Could you check a few things on this model? Use its own coordinates, in mm. Face numbers are marked on the shaded views. A direction names the side the tool comes from. Coordinates: 2 decimals unless noted, no trailing zeros. Loops run counter-clockwise (first coordinate to the right, second up) from the corner with the lowest first, then second, coordinate; pieces in that order, holes last. Notation, with made-up numbers: M 39,67 L 61,67 A21 cw 61,98 Z; hole C -20.5,-34 d5. An arc over 180 degrees is marked long. Write each question's results on one line, items separated by ' | '.
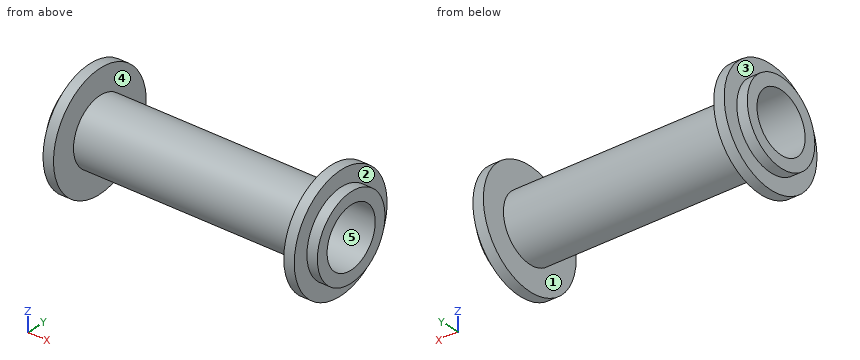
```python
from build123d import *

# Parameters (mm, degrees)
SKETCH2_R           = 5.7
CUT_EXTRUDE1_DEPTH  = 51.457903246
SKETCH3_R           = 8
SKETCH3_R_2         = 5.7
BOSS_EXTRUDE1_DEPTH = 2
SKETCH4_R           = 8
SKETCH4_R_2         = 5.7
BOSS_EXTRUDE2_DEPTH = 2


with BuildPart() as part:
    # Sketch1 → Revolve1 (revolve)
    with BuildSketch(Plane.XY, mode=Mode.PRIVATE) as revolve1_sk:
        Polygon((-24, 0), (24, 0), (24, 11), (22, 11), (22, 6.25), (-22, 6.25), (-22, 11), (-24, 11), align=None)
    revolve(revolve1_sk.sketch.rotate(Axis((-24, 0, 0), (1, 0, 0)), 180), axis=Axis((-24, 0, 0), (1, 0, 0)))

    # Sketch2 → Cut-Extrude1 (cut, through all)
    with BuildSketch(Plane(origin=(24, 0, 0), x_dir=(0, 0, -1), z_dir=(1, 0, 0))):
        Circle(SKETCH2_R)
    extrude(amount=-CUT_EXTRUDE1_DEPTH, mode=Mode.SUBTRACT)

    # Sketch3 → Boss-Extrude1 (add)
    with BuildSketch(Plane(origin=(24, 0, 0), x_dir=(0, 0, -1), z_dir=(1, 0, 0))):
        with Locations(Location((0, 0, 0), (0, 0, 270))):
            Circle(SKETCH3_R)
        Circle(SKETCH3_R_2, mode=Mode.SUBTRACT)
    extrude(amount=BOSS_EXTRUDE1_DEPTH)

    # Sketch4 → Boss-Extrude2 (add)
    with BuildSketch(Plane.ZY.offset(24)):
        with Locations(Location((0, 0, 0), (0, 0, 270))):
            Circle(SKETCH4_R)
        with Locations(Location((0, 0, 0), (0, 0, 180))):
            Circle(SKETCH4_R_2, mode=Mode.SUBTRACT)
    extrude(amount=BOSS_EXTRUDE2_DEPTH)


solid = part.part
```
(1) Will these pins go through, and if not, where does the flat tip stop? P1, Ø1, axis at x = -10, y = -5, coming from the -Z side; P2, Ø8, axis at x = -7, z = -6, coming from the +Y side; P3, Ø8, axis at x = -9.5, z = 7.5, coming from the +Y side.
Reported:
P1: stops at z = -4.34 | P2: stops at y = 5.92 | P3: stops at y = 5.18
(2) Imagine slicing it at C-C, the plane x = -15. List the corners of the cut face in (y, z) for me, and give its area (3 significant figures).
Reported:
outline: C 0,0 d12.5; hole C 0,0 d11.4 | area: 20.6 mm2
(3) Please list where these lines run through material, in increasing order: probe 1 along Z at (x, y) = (4, 0); probe 2 along X at (y, z) = (7.5, -3.5); probe 3 along Y at (x, z) = (-15, -0.5). Write a range as from..to.
Reported:
probe 1: z = -6.25..-5.7, 5.7..6.25 | probe 2: x = -24..-22, 22..24 | probe 3: y = -6.23..-5.68, 5.68..6.23
(4) Imagine slicing it at D-D, the plane y = -9. List the corners of the cut face in (x, z) for me.
Reported:
outline: M -24,-6.32 L -22,-6.32 L -22,6.32 L -24,6.32 Z; M 22,-6.32 L 24,-6.32 L 24,6.32 L 22,6.32 Z
(5) Which directions (+Z, -Z, +X, -X, +Y, -Y) give clear straight access to the entire face, cutting with the end or side of a thin tool? Please do the marked faces 1 and 2.
Reported:
face 1: none | face 2: +X
(6) If we mould it in two halves opening along X, with no side actions, what happens to the marked faces 3, 4 and 5? For each: released by +X, released by -X, zero draft, split by the parting line, or undercut.
Reported:
face 3: released by -X | face 4: undercut | face 5: zero draft
(7) Imagine slicing it at A-A, the plane z = 0. List the corners of the cut face in (x, y) for me.
Reported:
outline: M -26,-8 L -24,-8 L -24,-11 L -22,-11 L -22,-6.25 L 22,-6.25 L 22,-11 L 24,-11 L 24,-8 L 26,-8 L 26,-5.7 L -26,-5.7 Z; M -26,5.7 L 26,5.7 L 26,8 L 24,8 L 24,11 L 22,11 L 22,6.25 L -22,6.25 L -22,11 L -24,11 L -24,8 L -26,8 Z
